Read the model definition and answer for the solid it produces. Units are mm, in the model's axes. A direction names the side the tool comes from. Coordinates: 2 decimals unless noted, no trailing zeros. Write each loop counter-clockwise with the first axis right and the second up, starting at its lowest first coordinate (ties: lowest second). Pieces come first, ordered by that corner, then holes. Notation, with made-up numbers: (65.25, 81.25) -> (104.25, 81.25) arc R26 cw to (104.25, 111.25) -> close; hole circle Ø10 at (75, -14). An arc over 180 degrees is marked (long way). One line per item, written item: value. Start each with the question number.
1. Find section C-C, the plane z = 0. Write down the section's boundary in (x, y).
2. Given P1, Ø2.5, axis at y = 13, z = 65.5, coming from the -X side; P2, Ø3, axis at x = 0, z = -5, coming from the +Y side; P3, Ø12, axis at x = -41, z = -15, coming from the +Y side; P4, Ø9, axis at y = 9.5, z = 62, coming from the +X side, each flat-ended and moving along its own axis, determine where each tip first touches the part or whether it passes through.
3. Consider line 1 along X through (y, z) = (3.7, -5); line 2 along X through (y, z) = (26.5, 0); line 3 along Z through (x, y) = (35.5, 3.25). Determine where each line is inside the solid, lowest interval first.
4. Find section A-A, the plane x = 0. Write down the section's boundary in (y, z).
5. Find section B-B, the plane y = 16.5. Write down the section's boundary in (x, z), and give its area (3 significant figures).
6. For faces 4 (the cylindrical face through (39.369, 22.605, -42.934)), 5 (the flat face through (-6, 15, 64)), 6 (the flat face through (6, 15, 64)), 7 (the flat face through (0, 15, 68)), 8 (the flat face through (-60, 15, 1)), determine the directions among +Z, -Z, +X, -X, +Y, -Y from which every point of the face is accessible in a straight line to the end or side of a thin tool.
7. For a pull along Z with two mould halves and no side action, classify faces 1 (the flat face through (60, 15, 1)), 2 (the flat face through (33, 15, 60)), 3 (the flat face through (1, 5, -1)) as pulls with the +Z half, pulls with the -Z half, needs draft (parallel to the pull), parting line crosses it, or undercut.
```python
from build123d import *

# Parameters (mm, degrees)
SKETCH_1_W          = 120
SKETCH_1_H          = 120
EXTRUDE_1_DEPTH     = 30
SKETCH_2_R          = 58.25197646
CUT_EXTRUDE_1_DEPTH = 25
FILLET_1_R          = 10
SKETCH_3_R          = 2
CUT_EXTRUDE_2_DEPTH = 25
SKETCH_4_W          = 12
SKETCH_4_H          = 8
EXTRUDE_2_DEPTH     = 30


with BuildPart() as part:
    # 草图1 → 凸台-拉伸1 (new body)
    with BuildSketch(Plane(origin=(0, 0, 0), x_dir=(1, 0, 0), z_dir=(0, 1, 0))):
        Rectangle(SKETCH_1_W, SKETCH_1_H)
    extrude(amount=EXTRUDE_1_DEPTH)

    # 草图2 → 切除-拉伸1 (cut)
    with BuildSketch(Plane(origin=(0, 30, 0), x_dir=(1, 0, 0), z_dir=(0, 1, 0))):
        with Locations(Location((0, 0, 0), (0, 0, 270))):
            Circle(SKETCH_2_R)
    extrude(amount=-CUT_EXTRUDE_1_DEPTH, mode=Mode.SUBTRACT)

    # 圆角1
    fillet_1_edges = [part.edges().sort_by_distance(p)[0] for p in [
        (0, 5, -58.25197646),
    ]]
    fillet(fillet_1_edges, radius=FILLET_1_R)

    # 草图3 → 切除-拉伸2 (cut)
    with BuildSketch(Plane.XZ):
        with Locations(Location((0, -5, 0), (0, 0, 270))):
            Circle(SKETCH_3_R)
    extrude(amount=-CUT_EXTRUDE_2_DEPTH, mode=Mode.SUBTRACT)

    # 草图4 → 凸台-拉伸2 (add)
    with BuildSketch(Plane.XZ):
        with Locations((0, 64)):
            Rectangle(SKETCH_4_W, SKETCH_4_H)
    extrude(amount=-EXTRUDE_2_DEPTH)


solid = part.part
```
Answer block:
1. outline: (-60, 0) -> (60, 0) -> (60, 30) -> (58.25, 30) -> (58.25, 15) arc R10 cw to (48.25, 5) -> (-48.25, 5) arc R10 cw to (-58.25, 15) -> (-58.25, 30) -> (-60, 30) -> close
2. P1: stops at x = -6
2. P2: passes through
2. P3: stops at y = 5.1
2. P4: stops at x = 60
3. line 1: x = -60 to -2, 2 to 60
3. line 2: x = -60 to -58.25, 58.25 to 60
3. line 3: z = -60 to 60
4. outline: (0, -60) -> (30, -60) -> (30, -58.25) -> (15, -58.25) arc R10 cw to (5, -48.25) -> (5, -7) -> (0, -7) -> close; (0, -3) -> (5, -3) -> (5, 48.25) arc R10 cw to (15, 58.25) -> (30, 58.25) -> (30, 68) -> (0, 68) -> close
5. outline: (-60, -60) -> (60, -60) -> (60, 60) -> (6, 60) -> (6, 68) -> (-6, 68) -> (-6, 60) -> (-60, 60) -> close; hole circle Ø116.5 at (0, 0)
5. area: 3,840 mm2
6. face 4: +Y
6. face 5: +Z, -X, +Y, -Y
6. face 6: +Z, +X, +Y, -Y
6. face 7: +Z, +X, -X, +Y, -Y
6. face 8: +Z, -Z, -X, +Y, -Y
7. face 1: needs draft
7. face 2: pulls with the +Z half
7. face 3: undercut
